For this review, use the dimensioned drawing (mm, ordinates from the lowest corner) and the shaded views. A direction names the side the tool comes from. Coordinates: 2 decimals unless noted, no trailing zeros. Order: outer loops, then holes, each group sorted by start corner. A loop starts at its lowest first (then second) coordinate and runs counter-clockwise, first axis right, second up. Notation, with made-up numbers: M -30.75,41 L -13.75,41 A25 ccw -13.75,72 Z; hole C 62.5,-31 d3. An arc over 180 degrees is marked long. One line per item, written item: value.
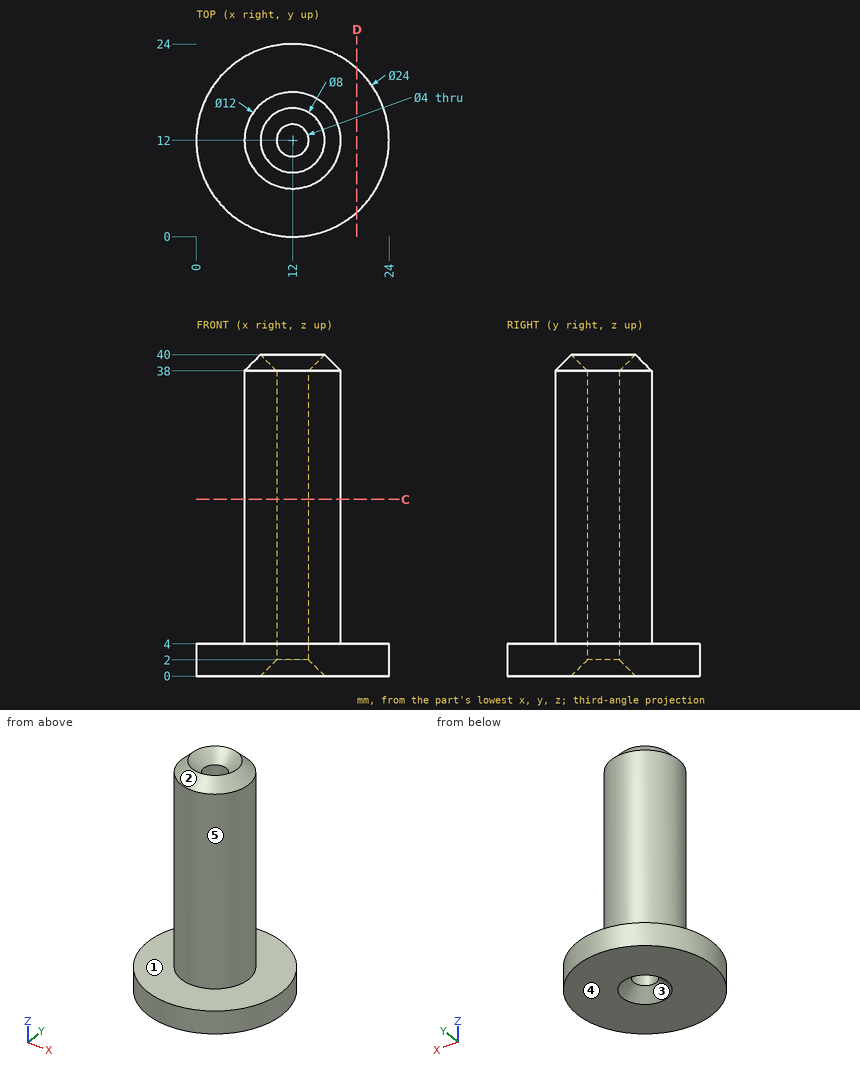
(1) For L1, parallel to Y at x = 12, z = 18.5; L2, parallel to Z at x = 11.25, y = 21.25; L3, parallel to X at y = 7.5, z = 23.5, list the stretches that pass through material, from the lowest coordinate up.
Geometry results:
L1: y = 6 to 10, 14 to 18
L2: z = 0 to 4
L3: x = 8.03 to 15.97
(2) We need section D-D, the plane x = 20. State the section outline as (y, z) points, plus the area to 3 significant figures.
Geometry results:
outline: M 3.06,0 L 20.94,0 L 20.94,4 L 3.06,4 Z
area: 71.6 mm2
(3) Tool access review of the marked faces 4 and 5: name each direction out of +Z, -Z, +X, -X, +Y, -Y from which nothing blocks a thin tool from reaching the whole face with its end or side.
Geometry results:
face 4: -Z, +X, -X, +Y, -Y
face 5: +Z
(4) Insertion check: pin 1 Ø1.5 at (x, y) = (15, 8.5) entering from +Z; pin 2 Ø1.5 at (x, y) = (17.5, 18) entering from +Z; pin 3 Ø4 at (x, z) = (11, 15.5) entering from +Y; pin 4 Ø4 at (x, z) = (7, 30) entering from -Y. Each pin has a flat end and moves straight along its axis. Give the tip position at first contact, or say it passes through.
Geometry results:
pin 1: stops at z = 40
pin 2: stops at z = 4
pin 3: stops at y = 18
pin 4: stops at y = 6.8
(5) We need section C-C, the plane z = 22. State the section outline as (x, y) points, plus the area to 3 significant figures.
Geometry results:
outline: C 12,12 d12; hole C 12,12 d4
area: 101 mm2
(6) Mouldability with a two-part tool opening along X and no side actions: class the marked faces 1, 2 and 3 as +X half, -X half, draft (parallel to the pull), parting line (faces both ways), or undercut.
Geometry results:
face 1: draft
face 2: parting line
face 3: undercut
